The model under review builds one solid part; all positions refer to its coordinate system, in mm. Coordinates: 2 decimals unless noted, no trailing zeros. Write each loop counter-clockwise with the first axis right and the second up, starting at its lowest first coordinate (ties: lowest second). Pieces come first, ordered by that corner, then holes. Notation, with made-up numbers: (75, 85.25) - (133, 85.25) arc R15 cw to (133, 108.25) - close; hole circle Ø9 at (-18, 45). An arc over 180 degrees is marked (long way). Put each result on its own line as item: value.
Solid Edge part; units mm, degrees
sketch "Sketch1" plane through (0, 0, 0) normal (0, 0, 1) x (1, 0, 0)
  line L0 (0, 0) -> (-165, 0)
  line L1 (-165, 0) -> (-165, -85.2)
  line L2 (-165, -85.2) -> (0, -85.2)
  line L3 (0, -85.2) -> (0, 0)
extrude "Protrusion1" add sketch "Sketch1" against normal blind 20
sketch "Sketch2" plane through (-82.5, -42.6, 0) normal (0, 0, 1) x (1, 0, 0)
  circle A0 centre (-42.5, -13.9) radius 6.65
  circle A1 centre (42.5, -13.9) radius 6.65
  circle A2 centre (-117.5, -6.9) radius 57.5
  circle A3 centre (117.5, -6.9) radius 57.5
extrude "ExtrudedCutout_1" cut sketch "Sketch2" against normal blind 20
chamfer "Chamfer_2" distance 1.8 angle 74 1 edges at (0, 0, -10) measured on face at (-25.85, 0, -16.4667)
chamfer "Chamfer_3" distance 1.8 angle 74 1 edges at (-165, 0, -10) measured on face at (-27.368, 0, -16.4667)
chamfer "Chamfer_4" distance 1.8 angle 74 1 edges at (-154.925, -85.2, -10) measured on face at (-132.2318, -85.2, -16.4667)
chamfer "Chamfer_5" distance 1.8 angle 74 1 edges at (-10.075, -85.2, -10) measured on face at (-130.7138, -85.2, -16.4667)
1. Consider section D-D on x = -149.5. State the section outline as (y, z) points, plus the area to 3 significant figures.
Determined:
outline: (-85.2, -20) - (-77, -20) - (-77, 0) - (-85.2, 0) - close; (-22, -20) - (0, -20) - (0, 0) - (-22, 0) - close
area: 604 mm^2
2. Consider section B-B on z = -6.25. State the section outline as (x, y) points, plus the area to 3 significant figures.
Determined:
outline: (-164.44, -4.32) arc R57.5 cw to (-153.62, -83.48) - (-153.12, -85.2) - (-11.88, -85.2) - (-11.38, -83.48) arc R57.5 cw to (-0.56, -4.32) - (-1.8, 0) - (-163.2, 0) - close; hole circle Ø13.3 at (-125, -56.5); hole circle Ø13.3 at (-40, -56.5)
area: 11,000 mm^2
3. Consider section A-A on x = -40. State the section outline as (y, z) points.
Determined:
outline: (-85.2, -20) - (-63.15, -20) - (-63.15, 0) - (-85.2, 0) - close; (-49.85, -20) - (0, -20) - (0, 0) - (-49.85, 0) - close
4. To check wall thickness, follow probe 1 along Y at (x, z) = (-125, -10); probe 2 along Y at (x, z) = (-37.5, -2.5); probe 3 along X at (y, z) = (-67, -11.5). State the ranges of each line that lie inside material, in increasing order.
Determined:
probe 1: y = -85.2 to -63.15, -49.85 to 0
probe 2: y = -85.2 to -62.66, -50.34 to 0
probe 3: x = -145.23 to -19.77
5. For pin 1 Ø6 at (y, z) = (-45, -6) entering from +X; pin 2 Ø8 at (y, z) = (-15, -10) entering from +X; pin 3 Ø4 at (y, z) = (-34.5, -10.5) entering from -X; pin 4 Ø12 at (x, y) = (-40, -56.5) entering from +Z, all flat-tipped, find the tip position at first contact; note any pin that passes through.
Determined:
pin 1: stops at x = -22.01
pin 2: stops at x = -7.71
pin 3: stops at x = -145.07
pin 4: passes through
6. Consider section C-C on y = -53.5. State the section outline as (x, z) points, plus the area to 3 significant figures.
Determined:
outline: (-142.64, -20) - (-130.93, -20) - (-130.93, 0) - (-142.64, 0) - close; (-119.07, -20) - (-45.93, -20) - (-45.93, 0) - (-119.07, 0) - close; (-34.07, -20) - (-22.36, -20) - (-22.36, 0) - (-34.07, 0) - close
area: 1,930 mm^2
7. The part is to be moulded in two halves that separate along Y. For faces 1 (the cylindrical face through (-21.883, -41.101, -9.86)), 2 (the flat face through (-163.81, -2.13, -9.86)), 3 (the cylindrical face through (-33.657, -54.503, -9.86)), 4 (the flat face through (-83, -85.2, -10)), say which applies: +Y half, -Y half, draft (parallel to the pull), parting line (faces both ways), or undercut.
Determined:
face 1: undercut
face 2: +Y half
face 3: undercut
face 4: -Y half
